Input: part model. Units: mm. Frame: model coordinates. A direction names the side the tool comes from. Round coordinates to 2 decimals unless told otherwise and drop trailing zeros. Loops run counter-clockwise (first coordinate to the right, second up) from the corner with the lowest first, then second, coordinate; pieces in that order, holes last. Notation, with made-up numbers: (-15, -37) -> (36, -37) arc R20 cw to (36, -31) -> close; hole circle Ø5 at (72.5, 11). An arc over 180 degrees is marked (long way). Answer in a Markdown table with one row per item. Add a question column.
Q1. Pin query (flat end, axial travel): pin 1 (0.8 mm diameter, centred on x = -27.5, z = 3.5, fed in from -Y); pin 2 (2 mm diameter, centred on x = -2.5, z = 2.5, fed in from -Y); pin 3 (0.8 mm diameter, centred on x = -28.5, z = 2.5, fed in from +Y). Return the tip coordinate at first contact, or that it passes through.
Q2. Ray query, L1, parallel to Y at x = -6.5, z = 5; L2, parallel to X at y = 9, z = 1.5; L3, parallel to X at y = -10, z = 5. Return the intervals inside material, ascending. Write a range as from..to.
Q3. Reachability of faces 1 (the face through (45.979, -21.097, 2.958)), 2 (the face through (-21.789, -3.843, 2.972)), 3 (the face through (-32.291, -5.778, 2.972)), 4 (the face through (-21.65, 3.767, 2.972)), 5 (the face through (35.971, 40.545, 2.958)) from +Z, -Z, +X, -X, +Y, -Y: full face, straight path, thin tool, end or side. Return the list, or none.
Q4. Section B-B, the plane x = -5.5. Output: boundary loops of the cut face in (y, z).
Q5. Section D-D, the plane y = 34. Output: boundary loops of the cut face in (x, z).
Q6. Section A-A, the plane x = 29. Output: boundary loops of the cut face in (y, z).
Autodesk Fusion 360 part; units mm, degrees
sketch "main" plane through (0, 0, 0) normal (0, 0, 1) x (1, 0, 0)
  circle A0 centre (21.8365, 0.0332) radius 2.25
  line L0 (-29.4135, 2.5332) -> (-26.9135, 2.5332)
  line L1 (-26.9135, -2.4668) -> (-29.4135, -2.4668)
  line L2 (-34.9258, 10.2857) -> (-33.9469, 12.3465) construction
  line L3 (-35.7535, 13.2046) -> (-36.7324, 11.1438)
  arc A1 (-32.9614, 14.0869) -> (-35.7535, 13.2046) centre (-33.9469, 12.3465) ccw
  arc A2 (-36.7324, 11.1438) -> (-35.9243, 8.5528) centre (-34.9258, 10.2857) ccw
  arc A3 (-24.2048, 6.0328) -> (-32.9614, 14.0869) centre (-45.9085, -8.7768) ccw
  line L4 (-36.7417, -11.0419) -> (-35.7592, -13.1001)
  arc A4 (-35.9295, -8.4441) -> (-36.7417, -11.0419) centre (-34.9367, -10.1804) ccw
  arc A5 (-35.7592, -13.1001) -> (-32.8186, -13.8848) centre (-33.9543, -12.2386) ccw
  line L5 (-32.8186, -13.8848) -> (-32.8147, -13.8915) construction
  arc A6 (-35.9295, -8.4441) -> (-29.4135, -2.4668) centre (-45.8569, 8.9181) ccw
  arc A7 (-26.9362, -2.4667) -> (-26.9135, 2.5332) centre (-26.9135, 0.0332) ccw
  arc A8 (-29.4135, 2.5332) -> (-35.9243, 8.5528) centre (-45.9085, -8.7768) ccw
  arc A9 (-26.9361, -2.4668) -> (-26.9362, -2.4667) centre (-45.9085, -8.7768) ccw
  arc A10 (-32.9737, -13.9817) -> (-24.2534, -6.0374) centre (-45.8569, 8.9181) ccw
  circle A11 centre (-18.4227, 9.9783) radius 7
  circle A12 centre (-18.498, -10.0217) radius 7
  line L6 (-18.4227, 2.9783) -> (17.5773, 2.9783)
  line L7 (-18.498, -3.0217) -> (17.502, -3.0217)
  line L8 (17.5773, 2.9783) -> (33.1079, 45.2119)
  line L9 (17.502, -3.0217) -> (33.4968, -34.2782)
  line L10 (47.9397, -21.8492) -> (36.7867, -34.6793)
  arc A13 (33.4968, -34.2782) -> (36.7867, -34.6793) centre (35.2773, -33.3672) ccw
  line L11 (47.9397, -21.8492) -> (43.9626, -20.3226)
  line L12 (43.9626, -20.3226) -> (37.3696, -27.907)
  line L13 (27.4111, -2.1643) -> (33.9251, -27.1004)
  arc A14 (33.9251, -27.1004) -> (37.3696, -27.907) centre (35.8602, -26.5949) ccw
  line L14 (27.2967, 2.403) -> (34.9624, 39.1928)
  arc A15 (27.2967, 2.403) -> (27.4111, -2.1643) centre (37.0865, 0.3632) ccw
  line L15 (37.7018, 40.6259) -> (47.9839, 36.2614)
  arc A16 (37.7018, 40.6259) -> (34.9624, 39.1928) centre (36.9204, 38.7849) ccw
  line L16 (47.9839, 36.2614) -> (47.421, 40.8458)
  line L17 (35.1018, 46.075) -> (47.421, 40.8458)
  arc A17 (35.1018, 46.075) -> (33.1079, 45.2119) centre (34.5157, 44.6942) ccw
  dimension "d1" = 5
  dimension "d3" = 4.5
  dimension "d4" = 2.5
  dimension "d5" = 40
  dimension "d6" = 40
  dimension "d7" = 4
  dimension "d9" = 4
  dimension "d11" = 52.55
  dimension "d12" = 52.55
  dimension "d13" = 4
  dimension "d14" = 4
  dimension "d15" = 14
  dimension "d16" = 14
  dimension "d17" = 20
  dimension "d20" = 110.19
  dimension "d22" = 117.1
  dimension "d25" = 68.1
  dimension "d26" = 2
  dimension "d27" = 17
  dimension "d28" = 4.26
  dimension "d29" = 70
  dimension "d30" = 110
  dimension "d31" = 55.64
  dimension "d32" = 2
  dimension "d33" = 153.59
  dimension "d34" = 10
  dimension "d35" = 78.77
  dimension "d36" = 2
  dimension "d37" = 11.17
  dimension "d38" = 60
  dimension "d39" = 120
  dimension "d40" = 4
  dimension "d41" = 1.5
  dimension "d45" = 48.75
  dimension "d47" = 15.25
  dimension "d48" = 36
  dimension "d49" = 6
extrude "Extrude1" add sketch "main" along normal blind 6 contours L0 L1 L3 A1 A2 A3 A7 A8 A9 A10 A11 A12 L6 L7 L8 L9 L10 A13 L11 L12 L13 A14 L14 A15 L15 A16 L16 L17 A17 | L1 L4 A4 A5 A6 A9 A10 picked at (-28.4657, -7.1435)
fillet "Fillet1" radius 1 28 edges at (-0.4227, 2.9783, 6) (-21.6924, 3.7889, 6) (-28.1213, 10.562, 6) (-34.5495, 14.2536, 6) (-36.2429, 12.1742, 6) (-36.8351, 9.6902, 6) (-32.3311, 5.9083, 6) (-32.337, -5.8201, 6) (-36.8456, -9.5835, 6) (-36.2504, -12.071, 6) (-34.5578, -14.1454, 6) (-28.1619, -10.5052, 6) (-21.7468, -3.8213, 6) (-0.498, -3.0217, 6) (-32.337, -5.8201, 0) (-36.8456, -9.5835, 0) (-36.2504, -12.071, 0) (-34.5578, -14.1454, 0) (-28.1619, -10.5052, 0) (-21.7468, -3.8213, 0) (-0.498, -3.0217, 0) (-0.4227, 2.9783, 0) (-21.6924, 3.7889, 0) (-28.1213, 10.562, 0) (-34.5495, 14.2536, 0) (-36.2429, 12.1742, 0) (-36.8351, 9.6902, 0) (-32.3311, 5.9083, 0)
equation "d47 = 13 mm + 2.25 mm"
Answer block:
| question | item | result |
|---|---|---|
| 1 | pin 1 | y = -10.26 |
| 1 | pin 2 | y = -3.02 |
| 1 | pin 3 | y = 11.25 |
| 2 | L1 | -3.02..2.98 |
| 2 | L2 | -36.46..-26.56, 19.79..28.67 |
| 2 | L3 | -36.93..-27.62, 21.07..29.46 |
| 3 | face 1 | +Z, -Z, +X |
| 3 | face 2 | +Z, -Z, -Y |
| 3 | face 3 | +Z, -Z, -X |
| 3 | face 4 | +Z, -Z, +Y |
| 3 | face 5 | +Z, -Z |
| 4 | outline | (-3.02, 1) arc R1 ccw to (-2.02, 0) -> (1.98, 0) arc R1 ccw to (2.98, 1) -> (2.98, 5) arc R1 ccw to (1.98, 6) -> (-2.02, 6) arc R1 ccw to (-3.02, 5) -> close |
| 5 | outline | (28.98, 0) -> (33.88, 0) -> (33.88, 6) -> (28.98, 6) -> close |
| 6 | outline | (-25.49, 0) -> (-8.25, 0) -> (-8.25, 6) -> (-25.49, 6) -> close; (10.58, 0) -> (34.04, 0) -> (34.04, 6) -> (10.58, 6) -> close |
